from build123d import *

# Parameters (mm, degrees)
BOSS_EXTRUDE1_DEPTH = 10
SKETCH2_W           = 78.14
SKETCH2_H           = 8.3
BOSS_EXTRUDE2_DEPTH = 60
SKETCH3_R           = 7.5
CUT_EXTRUDE1_DEPTH  = 10
FILLET1_R           = 5
CUT_EXTRUDE2_DEPTH  = 10
SKETCH5_R           = 2.5
BOSS_EXTRUDE3_DEPTH = 5
SKETCH7_R           = 1
CUT_EXTRUDE3_DEPTH  = 10


with BuildPart() as part:
    # Sketch1 → Boss-Extrude1 (new body)
    with BuildSketch(Plane.XY):
        Polygon((-104.14, 5), (-26, 5), (-26, -3.303087832), (-30.641562484, -3.303087832), (-40.234218738, -25), (-89.905781262, -25), (-99.498437516, -3.303087832), (-104.14, -3.303087832), align=None)
    extrude(amount=BOSS_EXTRUDE1_DEPTH)

    # Sketch2 → Boss-Extrude2 (add)
    with BuildSketch(Plane.XY.offset(10)):
        with Locations((-65.07, 0.85)):
            Rectangle(SKETCH2_W, SKETCH2_H)
    extrude(amount=BOSS_EXTRUDE2_DEPTH)

    # Sketch3 → Cut-Extrude1 (cut)
    with BuildSketch(Plane.XY.offset(10)):
        with Locations((-65.07, -13.5)):
            Circle(SKETCH3_R)
    extrude(amount=-CUT_EXTRUDE1_DEPTH, mode=Mode.SUBTRACT)

    # Fillet1
    fillet1_edges = [part.edges().sort_by_distance(p)[0] for p in [
        (-26, 0.848456084, 0),
        (-104.14, 0.848456084, 0),
    ]]
    fillet(fillet1_edges, radius=FILLET1_R)

    # Sketch4 → Cut-Extrude2 (cut)
    with BuildSketch(Plane.XZ.offset(3.3)):
        Polygon((-84.531238134, 70), (-104.14, 42.355810036), (-104.14, 70), align=None)
        Polygon((-45.608761866, 70), (-26, 42.355810036), (-26, 70), align=None)
    extrude(amount=-CUT_EXTRUDE2_DEPTH, mode=Mode.SUBTRACT)

    # Sketch5 → Boss-Extrude3 (add)
    with BuildSketch(Plane.XZ.offset(3.3)):
        with Locations(Location((-85.07, 38, 0), (0, 0, 90))):
            Circle(SKETCH5_R)
        with Locations(Location((-45.07, 38, 0), (0, 0, 90))):
            Circle(SKETCH5_R)
    boss_extrude3 = extrude(amount=BOSS_EXTRUDE3_DEPTH)

    # Mirror1: Boss-Extrude3 across plane
    add(boss_extrude3.mirror(Plane.ZX))

    # Sketch7 → Cut-Extrude3 (cut)
    with BuildSketch(Plane.XZ.offset(3.3)):
        with Locations(Location((-60.07, 64.945333525, 0), (0, 0, 270))):
            Circle(SKETCH7_R)
        with Locations(Location((-70.07, 64.945333525, 0), (0, 0, 270))):
            Circle(SKETCH7_R)
    extrude(amount=-CUT_EXTRUDE3_DEPTH, mode=Mode.SUBTRACT)


solid = part.part
For this review, take the finished solid that the model builds, in its own axes (mm). A direction names the side the tool comes from. Round coordinates to 2 decimals unless told otherwise and drop trailing zeros. Loops run counter-clockwise (first coordinate to the right, second up) from the corner with the lowest first, then second, coordinate; pieces in that order, holes last. Notation, with made-up numbers: (-0.75, 67.5) - (24.25, 67.5) arc R17 ccw to (24.25, 75.5) - close; hole circle Ø5 at (6, 60.5). An arc over 180 degrees is marked (long way). One line per item, written item: value. Start each with the question number.
Item 1: The part is to be moulded in two halves that separate along X. For faces 1 (the cylindrical face through (-45.821, 6.627, 40.385)), 2 (the flat face through (-35.37, -14, 4.93)), 3 (the flat face through (-104.14, 1, 23)), 4 (the flat face through (-64.5, -21.2, 10)), say which applies: +X half, -X half, draft (parallel to the pull), parting line (faces both ways), or undercut.
Item 2: Clearance check with flat-ended pins moving along their axes: pin 1 Ø5 at (x, z) = (-27.5, 3) entering from -Y; pin 2 Ø13.5 at (x, y) = (-65.07, -13.5) entering from +Z; pin 3 Ø6.5 at (x, y) = (-81.5, -11.5) entering from +Z; pin 4 Ø5 at (x, z) = (-73, 58.5) entering from +Y. State where each tip first meets the part, or that it passes through.
Item 3: Take a section at B-B (y = 2). Give the boundary of the cut face in (x, z), plus the area to 3 significant figures.
Item 4: For L1, parallel to Y at x = -65.07, z = 2.5; L2, parallel to Z at x = -60, y = 1; L3, parallel to Z at x = -48, y = -18, list the stretches that pass through material, from the lowest coordinate up.
Item 5: Take a section at A-A (x = -65.07). Give the boundary of the cut face in (y, z).
Item 6: Take a section at D-D (y = -13.5). Give the boundary of the cut face in (x, z).
Item 7: Take a section at C-C (z = 8.5). Give the boundary of the cut face in (x, y), plus the area to 3 significant figures.
Item 8: For faces 5 (the flat face through (-85, -8.3, 38)), 6 (the flat face through (-102, -3.303, 5)), 7 (the flat face through (-28, -3.303, 5)), 8 (the cylindrical face through (-82.85, 6.63, 39.15)), list the 3-axis set-ups (+Z, -Z, +X, -X, +Y, -Y) from which the entire face can be reached by the end or side of a thin tool; tool diameter is ignored.
Answer below:
1. face 1: undercut
1. face 2: +X half
1. face 3: -X half
1. face 4: draft
2. pin 1: stops at y = -3.3
2. pin 2: passes through
2. pin 3: stops at z = 10
2. pin 4: stops at y = 5
3. outline: (-104.14, 5) arc R5 ccw to (-99.14, 0) - (-31, 0) arc R5 ccw to (-26, 5) - (-26, 42.36) - (-45.61, 70) - (-84.53, 70) - (-104.14, 42.36) - close; hole circle Ø2 at (-70.07, 64.95); hole circle Ø2 at (-60.07, 64.95)
3. area: 4,910 mm2
4. L1: y = -25 to -21, -6 to 5
4. L2: z = 0 to 63.95, 65.94 to 70
4. L3: z = 0 to 10
5. outline: (-25, 0) - (-21, 0) - (-21, 10) - (-25, 10) - close; (-6, 0) - (5, 0) - (5, 70) - (-3.3, 70) - (-3.3, 10) - (-6, 10) - close
6. outline: (-94.99, 0) - (-72.57, 0) - (-72.57, 10) - (-94.99, 10) - close; (-57.57, 0) - (-35.15, 0) - (-35.15, 10) - (-57.57, 10) - close
7. outline: (-104.14, -3.3) - (-99.5, -3.3) - (-89.91, -25) - (-40.23, -25) - (-30.64, -3.3) - (-26, -3.3) - (-26, 5) - (-104.14, 5) - close; hole circle Ø15 at (-65.07, -13.5)
7. area: 1,760 mm2
8. face 5: +Z, +X, -X, -Y
8. face 6: +Z, -Z, -X, -Y
8. face 7: +Z, -Z, +X, -Y
8. face 8: +Y
